Check sheet for the drawn part. Datum: minimum x, y, z corner. Units: mm. Coordinates: 2 decimals unless noted, no trailing zeros. Order: outer loops, then holes, each group sorted by start corner. A loop starts at its lowest first (then second) coordinate and runs counter-clockwise, first axis right, second up. Notation, with made-up numbers: (88.25, 55) - (96.25, 55) arc R14 ccw to (96.25, 81) - close; hole circle Ø2 at (73, -0.5). An arc over 180 degrees is marked (long way). Put each result on its own line as item: value.
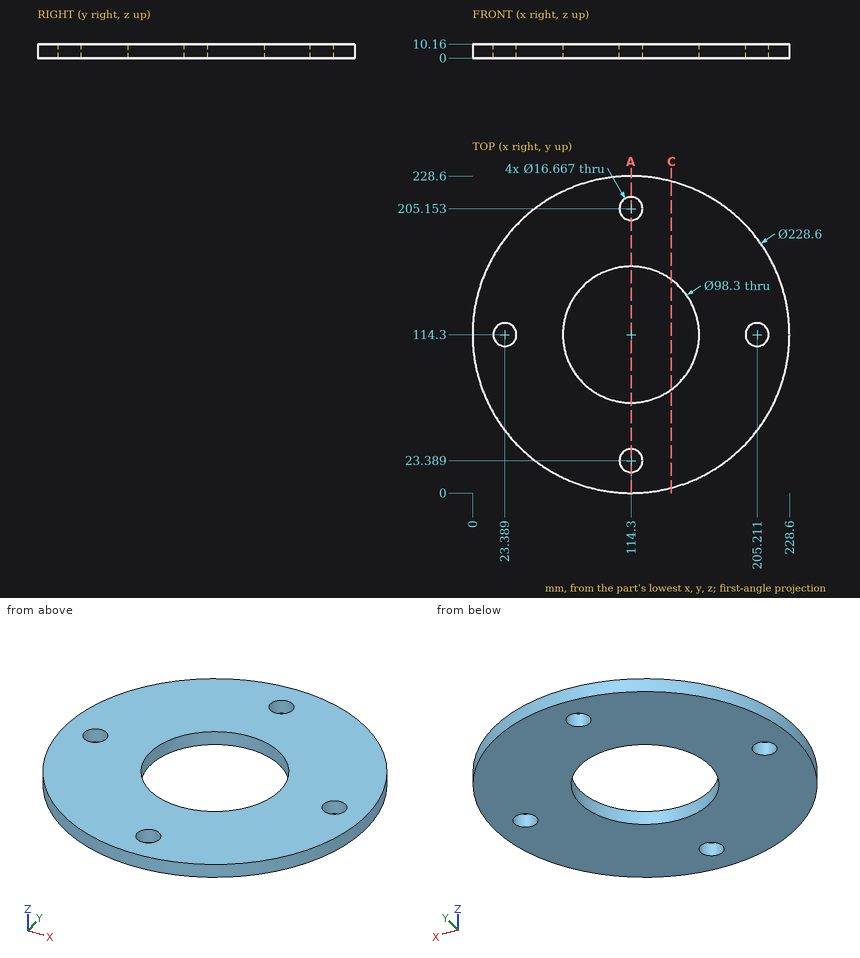
Q1. Thickness scan on L1, parallel to X at y = 114, z = 1.75; L2, parallel to X at y = 121, z = 9.75 (1 decimal); L3, parallel to Y at x = 131, z = 2.25 (1 decimal). Record the ranges inside material, lowest first. Write a range as [from, to].
Answer block:
L1: x = [0, 15.06], [31.72, 65.15], [163.45, 196.88], [213.54, 228.6]
L2: x = [0.2, 18.4], [28.3, 65.6], [163, 200.3], [210.2, 228.4]
L3: y = [1.2, 68.1], [160.5, 227.4]
Q2. Section check C-C on x = 143.5. Record the boundary of the cut face in (y, z) (1 decimal).
Answer block:
outline: (3.8, 0) - (74.8, 0) - (74.8, 10.2) - (3.8, 10.2) - close; (153.8, 0) - (224.8, 0) - (224.8, 10.2) - (153.8, 10.2) - close
Q3. Section check A-A on x = 114.3. State how many separate pieces and enclosed holes the cut face has, then the cut area to 3 significant figures.
Answer block:
separate pieces: 4
enclosed holes: 0
area: 985 mm^2
Q4. Depth check by flat-ended pin: pin 1 Ø5 at (x, z) = (140, 4) entering from +Y; pin 2 Ø1.5 at (x, z) = (153.5, 5.5) entering from -Y; pin 3 Ø1.5 at (y, z) = (56, 2.5) entering from +X (1 decimal). Enter the tip coordinate at first touch or a pass-through.
Answer block:
pin 1: stops at y = 226.22
pin 2: stops at y = 6.66
pin 3: stops at x = 213.1
